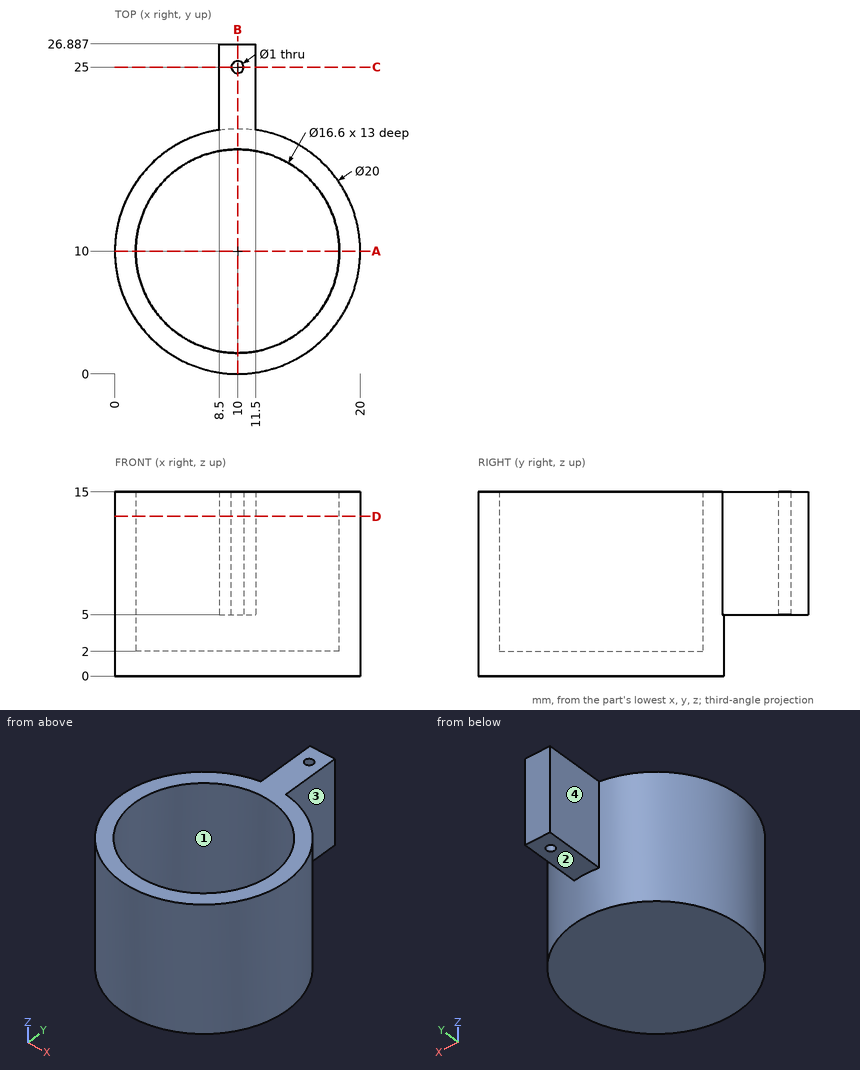
For this review, use the dimensioned drawing (mm, ordinates from the lowest corner) and the shaded views. Coordinates: 2 decimals unless noted, no trailing zeros. Order: outer loops, then holes, each group sorted by start corner. A loop starts at its lowest first (then second) coordinate and runs counter-clockwise, first axis right, second up. Notation, with made-up numbers: (-26.5, -36) -> (12.5, -36) arc R24 cw to (12.5, -23) -> close; hole circle Ø3 at (-29, 70). An arc over 180 degrees is marked (long way). One line per item, written item: value. Start each with the question number.
Q1. Take a section at B-B, the plane x = 10. State the section outline as (y, z) points, then the cut area to 3 significant figures.
Q2. Mouldability with a two-part tool opening along X and no side actions: class the marked faces 1, 2, 3 and 4 as pulls with the +X half, pulls with the -X half, needs draft (parallel to the pull), parting line crosses it, or undercut.
Q3. Take a section at D-D, the plane z = 13. State the section outline as (x, y) points, then the cut area to 3 significant figures.
Q4. Insertion check: pin 1 Ø4 at (y, z) = (6.5, 8.5) entering from -X; pin 2 Ø1.5 at (x, y) = (10, 25) entering from -Z; pin 3 Ø2 at (y, z) = (22.5, 12.5) entering from -X. Each pin has a flat end and moves straight along its axis. Give the tip position at first contact, or say it passes through.
Q5. Take a section at C-C, the plane y = 25. State the section outline as (x, z) points.
Q6. For probe 1 along Y at (x, z) = (10, 7); probe 2 along X at (y, z) = (10.25, 7); probe 3 along X at (y, z) = (25, 10), list the stretches that pass through material, from the lowest coordinate up.
Q7. Take a section at A-A, the plane y = 10. State the section outline as (x, z) points.
Values follow:
1. outline: (0, 0) -> (20, 0) -> (20, 5) -> (24.5, 5) -> (24.5, 15) -> (18.3, 15) -> (18.3, 2) -> (1.7, 2) -> (1.7, 15) -> (0, 15) -> close; (25.5, 5) -> (26.89, 5) -> (26.89, 15) -> (25.5, 15) -> close
1. area: 143 mm2
2. face 1: undercut
2. face 2: needs draft
2. face 3: pulls with the +X half
2. face 4: pulls with the -X half
3. outline: (8.5, 19.89) arc R10 ccw (long way) to (11.5, 19.89) -> (11.5, 26.89) -> (8.5, 26.89) -> close; hole circle Ø16.6 at (10, 10); hole circle Ø1 at (10, 25)
3. area: 118 mm2
4. pin 1: stops at x = 0.11
4. pin 2: stops at z = 5
4. pin 3: stops at x = 8.5
5. outline: (8.5, 5) -> (9.5, 5) -> (9.5, 15) -> (8.5, 15) -> close; (10.5, 5) -> (11.5, 5) -> (11.5, 15) -> (10.5, 15) -> close
6. probe 1: y = 0 to 1.7, 18.3 to 24.5, 25.5 to 26.89
6. probe 2: x = 0 to 1.7, 18.3 to 20
6. probe 3: x = 8.5 to 9.5, 10.5 to 11.5
7. outline: (0, 0) -> (20, 0) -> (20, 15) -> (18.3, 15) -> (18.3, 2) -> (1.7, 2) -> (1.7, 15) -> (0, 15) -> close
